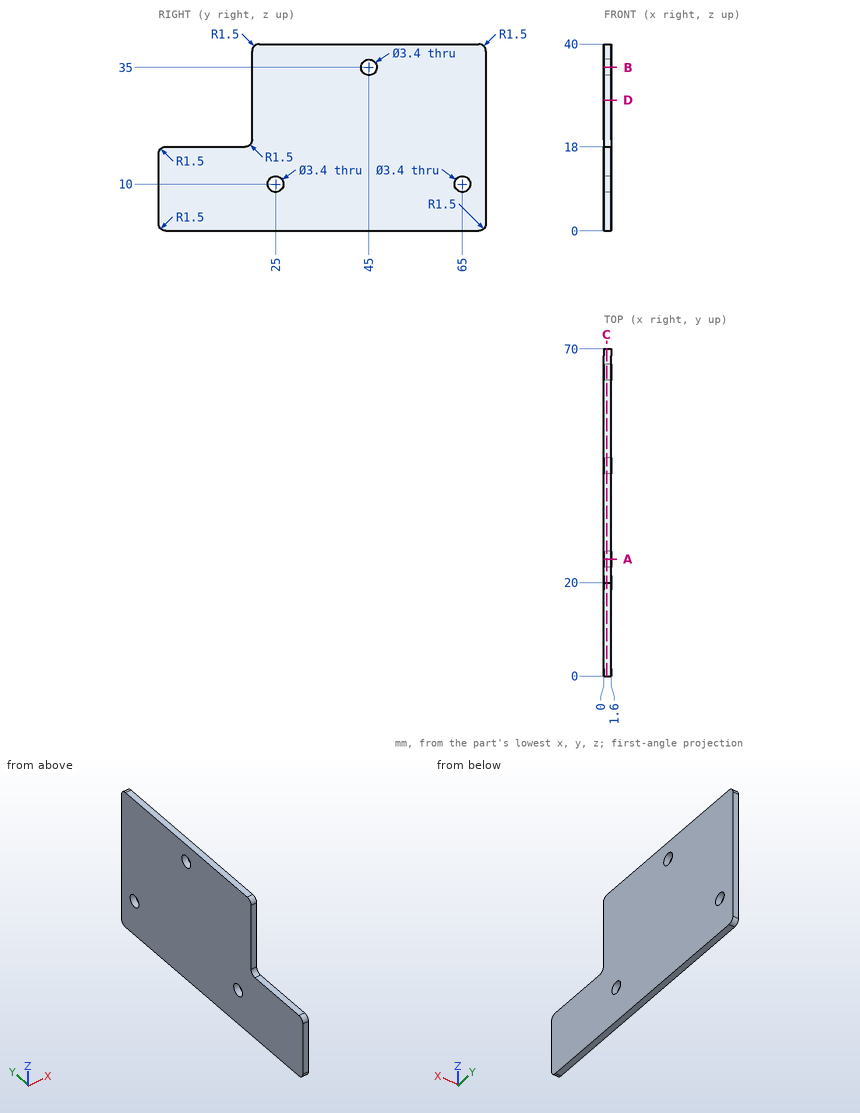
The drawing under review shows one solid part. Ordinate dimensions are in mm from its lowest x, y, z. Coordinates: 2 decimals unless noted, no trailing zeros. Loops run counter-clockwise (first coordinate to the right, second up) from the corner with the lowest first, then second, coordinate; pieces in that order, holes last. Notation, with made-up numbers: M 22.25,-15 L 61.25,-15 A15 ccw 61.25,7 Z; hole C 2.5,43 d3. An arc over 180 degrees is marked long. Use one line per item in the form item = value.
(1) Consider section A-A (y = 25). Write out the cut boundary in (x, z).
Return value:
outline = M 0,0 L 1.6,0 L 1.6,8.3 L 0,8.3 Z; M 0,11.7 L 1.6,11.7 L 1.6,40 L 0,40 Z
(2) Consider section C-C (x = 0.6). Write out the cut boundary in (y, z).
Return value:
outline = M 0,1.5 A1.5 ccw 1.5,0 L 68.5,0 A1.5 ccw 70,1.5 L 70,38.5 A1.5 ccw 68.5,40 L 21.5,40 A1.5 ccw 20,38.5 L 20,19.5 A1.5 cw 18.5,18 L 1.5,18 A1.5 ccw 0,16.5 Z; hole C 25,10 d3.4; hole C 45,35 d3.4; hole C 65,10 d3.4
(3) Consider section D-D (z = 28). Write out the cut boundary in (x, y).
Return value:
outline = M 0,20 L 1.6,20 L 1.6,70 L 0,70 Z
(4) Clearance check with a flat-ended pin moving along its axis: P1, Ø0.8, axis at x = 1, z = 29.5, coming from the -Y side. State where the tip first meets the part, or that it passes through.
Return value:
P1 = 20
(5) Consider section B-B (z = 35). Write out the cut boundary in (x, y).
Return value:
outline = M 0,20 L 1.6,20 L 1.6,43.3 L 0,43.3 Z; M 0,46.7 L 1.6,46.7 L 1.6,70 L 0,70 Z
(6) For line 1 along Y through (x, z) = (0.6, 10); line 2 along Z through (x, y) = (0.9, 65); line 3 along Y through (x, z) = (0.95, 35), list the stretches that pass through material, from the lowest coordinate up. Write a range as from..to.
Return value:
line_1 = 0..23.3, 26.7..63.3, 66.7..70
line_2 = 0..8.3, 11.7..40
line_3 = 20..43.3, 46.7..70
